```python
from build123d import *

# Parameters (mm, degrees)
ESBO_O1_R                = 21
RESSALTO_EXTRUS_O1_DEPTH = 15
ESBO_O2_R                = 6.5
RESSALTO_EXTRUS_O2_DEPTH = 65
CHANFRO1_SIZE            = 15
CHANFRO1_SIZE2           = 6.213203436
ESBO_O3_R                = 2.5
CORTE_EXTRUS_O2_DEPTH    = 4000
ESBO_O3_3_R              = 4.5
ESBO_O3_3_R_2            = 2.5
ESBO_O3_3_R_3            = 3.749939631
CORTE_EXTRUS_O3_DEPTH    = 6


with BuildPart() as part:
    # Esbo_o1 → Ressalto-extrus_o1 (new body)
    with BuildSketch(Plane(origin=(470, 0, 0), x_dir=(0, 0, -1), z_dir=(1, 0, 0))):
        with Locations((-750, 0)):
            Circle(ESBO_O1_R)
    extrude(amount=RESSALTO_EXTRUS_O1_DEPTH)

    # Esbo_o2 → Ressalto-extrus_o2 (add)
    with BuildSketch(Plane(origin=(485, 0, 0), x_dir=(0, 0, -1), z_dir=(1, 0, 0))):
        with Locations((-750, 0)):
            Circle(ESBO_O2_R)
    extrude(amount=RESSALTO_EXTRUS_O2_DEPTH)

    # Chanfro1
    chanfro1_edges = [part.edges().sort_by_distance(p)[0] for p in [
        (550, 0, 756.5),
    ]]
    chanfro1_side = [part.faces().sort_by_distance(p)[0] for p in [
        (517.5, 0, 756.5),
    ]]
    chamfer(chanfro1_edges, length=CHANFRO1_SIZE, length2=CHANFRO1_SIZE2, reference=chanfro1_side[0])

    # Esbo_o3 → Corte-extrus_o2 (cut)
    with BuildSketch(Plane(origin=(485, 0, 0), x_dir=(0, 0, -1), z_dir=(1, 0, 0))):
        with Locations((-738.884845661, 11.158666767)):
            Circle(ESBO_O3_R)
        with Locations((-734.250030053, 0.030767933)):
            Circle(ESBO_O3_R)
        with Locations((-738.841333233, -11.115154339)):
            Circle(ESBO_O3_R)
        with Locations((-749.969232067, -15.749969947)):
            Circle(ESBO_O3_R)
        with Locations((-761.115154339, -11.158666767)):
            Circle(ESBO_O3_R)
        with Locations((-765.749969947, -0.030767933)):
            Circle(ESBO_O3_R)
        with Locations((-761.158666767, 11.115154339)):
            Circle(ESBO_O3_R)
        with Locations((-750.030767933, 15.749969947)):
            Circle(ESBO_O3_R)
    extrude(amount=-CORTE_EXTRUS_O2_DEPTH, mode=Mode.SUBTRACT)

    # Esbo_o3_3 → Corte-extrus_o3 (cut)
    with BuildSketch(Plane(origin=(485, 0, 0), x_dir=(0, 0, -1), z_dir=(1, 0, 0))):
        with Locations((-750.070911646, 15.833410446)):
            Circle(ESBO_O3_3_R)
        with Locations((-750.030767933, 15.749969947)):
            Circle(ESBO_O3_3_R_2, mode=Mode.SUBTRACT)
        with Locations((-738.890427188, 11.258735336)):
            Circle(ESBO_O3_3_R)
        with Locations((-738.884845661, 11.158666767)):
            Circle(ESBO_O3_3_R_2, mode=Mode.SUBTRACT)
        with Locations((-734.219414603, 0.118155167)):
            Circle(ESBO_O3_3_R)
        with Locations((-734.250030053, 0.030767933)):
            Circle(ESBO_O3_3_R_2, mode=Mode.SUBTRACT)
        with Locations((-738.794089712, -11.062329291)):
            Circle(ESBO_O3_3_R)
        with Locations((-738.841333233, -11.115154339)):
            Circle(ESBO_O3_3_R_2, mode=Mode.SUBTRACT)
        with Locations((-749.934669881, -15.733341876)):
            Circle(ESBO_O3_3_R)
        with Locations((-749.969232067, -15.749969947)):
            Circle(ESBO_O3_3_R_2, mode=Mode.SUBTRACT)
        with Locations((-761.115154339, -11.158666767)):
            Circle(ESBO_O3_3_R)
        with Locations((-761.115154339, -11.158666767)):
            Circle(ESBO_O3_3_R_2, mode=Mode.SUBTRACT)
        with Locations((-765.786166925, -0.018086598)):
            Circle(ESBO_O3_3_R)
        with Locations((-765.749969947, -0.030767933)):
            Circle(ESBO_O3_3_R_3, mode=Mode.SUBTRACT)
        with Locations((-765.749969947, -0.030767933)):
            Circle(ESBO_O3_3_R_3)
        with Locations((-765.749969947, -0.030767933)):
            Circle(ESBO_O3_3_R_2, mode=Mode.SUBTRACT)
        with Locations((-761.211491815, 11.16239786)):
            Circle(ESBO_O3_3_R)
        with Locations((-761.158666767, 11.115154339)):
            Circle(ESBO_O3_3_R_2, mode=Mode.SUBTRACT)
    extrude(amount=-CORTE_EXTRUS_O3_DEPTH, mode=Mode.SUBTRACT)


solid = part.part
```
Geometry check sheet. Reference: the model listing, model coordinates, mm. A direction names the side the tool comes from. Give positions to 0.01 mm unless a question says otherwise; leave off trailing zeros. Order: outer loops, then holes, each group sorted by start corner. A loop starts at its lowest first (then second) coordinate and runs counter-clockwise, first axis right, second up. Notation, with made-up numbers: (-28, 37.5) - (-1, 37.5) arc R14 ccw to (-1, 44.5) - close; hole circle Ø3 at (85, 81). An arc over 180 degrees is marked (long way). Answer in a Markdown table with one row per item. Add a question column.
Q1. Cross-section at A-A, the plane x = 483.5. Count the separate pieces of the cut face and the enclosed holes in it, then the cut area to 3 significant figures.
Q2. Cross-section at B-B, the plane x = 510. Enter the section's corners in (y, z).
Q3. Mould release check, pull along Z, two halves, no side actions. Record for faces 3 (the flat face through (485, 5, 745.6)), 4 (the cylindrical face through (474.563, -13.377, 759.962)), 5 (the conical face through (544.272, 0.117, 752.657)): pulls with the +Z half, pulls with the -Z half, needs draft (parallel to the pull), parting line crosses it, or undercut.
Q4. Material ranges on probe 1 along Y at (x, z) = (481.5, 747.5); probe 2 along X at (y, z) = (-10.5, 748); probe 3 along X at (y, z) = (-12.5, 749), recorded low to high. Write a range as from..to.
Q5. Cross-section at C-C, the plane x = 536.5. Enter the section's corners in (y, z).
Q6. Gauge pin test, flat ends, axial feed: pin 1 (4.5 mm diameter, centred on y = -11.16, z = 761.12, fed in from +X); pin 2 (10 mm diameter, centred on y = -18, z = 750.5, fed in from +X); pin 3 (7 mm diameter, centred on y = 15.83, z = 750.07, fed in from -X); pin 4 (6 mm diameter, centred on y = -0.03, z = 765.75, fed in from +X). Record the tip position at first contact, or that the pin passes through.
Q7. Tool access check on faces 1 (the cylindrical face through (509.65, 0.286, 756.494)), 2 (the cylindrical face through (474.56, -16.71, 747.66)). Record the directions out of +Z, -Z, +X, -X, +Y, -Y that give a thin tool (end or side, any length) a straight path to the whole face; none if there is none.
Check values:
| question | item | result |
|---|---|---|
| 1 | separate pieces | 1 |
| 1 | enclosed holes | 8 |
| 1 | area | 877 mm^2 |
| 2 | outline | circle Ø13 at (0, 750) |
| 3 | face 3 | needs draft |
| 3 | face 4 | undercut |
| 3 | face 5 | parting line crosses it |
| 4 | probe 1 | y = -20.85..-19.52, -11.95..12.14, 19.53..20.85 |
| 4 | probe 2 | x = 470..485 |
| 4 | probe 3 | x = 470..479 |
| 5 | outline | circle Ø11.76 at (0, 750) |
| 6 | pin 1 | passes through |
| 6 | pin 2 | stops at x = 485 |
| 6 | pin 3 | stops at x = 470 |
| 6 | pin 4 | stops at x = 479 |
| 7 | face 1 | +X |
| 7 | face 2 | +X, -X |
